Part model, mm, in its own coordinate system. A direction names the side the tool comes from. Round coordinates to 2 decimals unless told otherwise and drop trailing zeros. Write each loop counter-clockwise with the first axis right and the second up, starting at its lowest first coordinate (ties: lowest second). Pieces come first, ordered by that corner, then holes. Notation, with made-up numbers: (-14, -6.5) -> (1, -6.5) arc R21 ccw to (1, 23.5) -> close; hole circle Ø8 at (70, 79). An arc over 180 degrees is marked (long way). Return JSON: item names as keys, results as strings. Group by question number.
```python
from build123d import *

# Parameters (mm, degrees)
SZKIC4_R                    = 75
DODANIE_WYCI_GNI_CIE2_DEPTH = 14
SZKIC5_R                    = 23.5
WYTNIJ_WYCI_GNI_CIE3_DEPTH  = 12
SZKIC6_R                    = 13
WYTNIJ_WYCI_GNI_CIE4_DEPTH  = 12
SZKIC7_R                    = 75
SZKIC7_R_2                  = 72.5
WYTNIJ_WYCI_GNI_CIE5_DEPTH  = 10
SZKIC8_R                    = 1.5
WYTNIJ_WYCI_GNI_CIE6_DEPTH  = 6
SZKIC10_R                   = 1.5
WYTNIJ_WYCI_GNI_CIE7_DEPTH  = 6
SZYK_KO_OWY1_COUNT          = 4


with BuildPart() as part:
    # Szkic4 → Dodanie-wyciągnięcie2 (new body)
    with BuildSketch(Plane(origin=(0, 0, 0), x_dir=(1, 0, 0), z_dir=(0, 1, 0))):
        Circle(SZKIC4_R)
    extrude(amount=DODANIE_WYCI_GNI_CIE2_DEPTH)

    # Szkic5 → Wytnij-wyciągnięcie3 (cut)
    with BuildSketch(Plane(origin=(0, 14, 0), x_dir=(1, 0, 0), z_dir=(0, 1, 0))):
        Circle(SZKIC5_R)
    extrude(amount=-WYTNIJ_WYCI_GNI_CIE3_DEPTH, mode=Mode.SUBTRACT)

    # Szkic6 → Wytnij-wyciągnięcie4 (cut)
    with BuildSketch(Plane(origin=(0, 2, 0), x_dir=(1, 0, 0), z_dir=(0, 1, 0))):
        Circle(SZKIC6_R)
    extrude(amount=-WYTNIJ_WYCI_GNI_CIE4_DEPTH, mode=Mode.SUBTRACT)

    # Szkic7 → Wytnij-wyciągnięcie5 (cut)
    with BuildSketch(Plane.XZ):
        Circle(SZKIC7_R)
        Circle(SZKIC7_R_2, mode=Mode.SUBTRACT)
    extrude(amount=-WYTNIJ_WYCI_GNI_CIE5_DEPTH, mode=Mode.SUBTRACT)

    # Szkic8 → Wytnij-wyciągnięcie6 (cut)
    with BuildSketch(Plane(origin=(0, 0, 0), x_dir=(-1, 0, 0), z_dir=(0, -1, 0))):
        with Locations((23.060270904, -19.500356556)):
            Circle(SZKIC8_R)
        with Locations((-28.863517887, 24.407731054)):
            Circle(SZKIC8_R)
    extrude(amount=-WYTNIJ_WYCI_GNI_CIE6_DEPTH, mode=Mode.SUBTRACT)

    # Szkic10 → Wytnij-wyciągnięcie7 (cut)
    with BuildSketch(Plane(origin=(0, 0, 72.5), x_dir=(0, -1, 0), z_dir=(0, 0, -1))):
        with Locations((-6, 6)):
            Circle(SZKIC10_R)
    wytnij_wyci_gni_cie7 = extrude(amount=WYTNIJ_WYCI_GNI_CIE7_DEPTH, mode=Mode.SUBTRACT)

    # Szyk kołowy1: Wytnij-wyciągnięcie7 ×4 about axis
    szyk_ko_owy1_axis = Axis((0, 0, 0), (0, 1, 0))
    for i in range(1, SZYK_KO_OWY1_COUNT):
        add(wytnij_wyci_gni_cie7.rotate(szyk_ko_owy1_axis, i * 360 / SZYK_KO_OWY1_COUNT), mode=Mode.SUBTRACT)


solid = part.part
```
Item 1: Wall check: L1, parallel to X at y = 5.25, z = -1; L2, parallel to Y at x = 67, z = -31; L3, parallel to Z at x = -1, y = 12.5. Give the ranges that are in metal, low to high.
Item 2: Two-plate mould, pull along X, no slides. Class faces 1 (the face through (-10.316, 1.014, 7.91)), 2 (the face through (69.15, 4.93, 21.78)), 3 (the face through (-39.2, 10, 61.5)): released by +X, released by -X, zero draft, split by the parting line, or undercut.
Item 3: Cut at B-B (z = 0). Write the cut outline in (x, y), then the cut area to 3 significant figures.
Item 4: Flat gauge pins, fed straight in: P1, Ø2.5, axis at y = 6, z = 6, coming from the -X side; P2, Ø5, axis at y = 9, z = 26.5, coming from the +X side; P3, Ø8, axis at x = 13, z = -10.5, coming from the +Y side. Where does each tip first touch, or does it go through?
Item 5: Cut at C-C (z = -28). Write the cut outline in (x, y), then the cut area to 3 significant figures.
Item 6: Which spindle directions (+Z, -Z, +X, -X, +Y, -Y) get a long thin tool onto all of the face, cutting with end or side? Do faces 4 (the face through (22.4, 8.1, -7.1)), 5 (the face through (16, 14, -18)). Say none if no direction does.
Item 7: Cut at D-D (x = 44). Write the cut outline in (y, z), then the cut area to 3 significant figures.
Item 8: Cut at A-A (x = 0). Write the cut outline in (y, z), then the cut area to 3 significant figures.
Checks:
{
 "1": {"L1": "x = -72.49 to -23.48, 23.48 to 72.49", "L2": "y = 10 to 14", "L3": "z = -74.99 to -23.48, 23.48 to 74.99"},
 "2": {"face 1": "undercut", "face 2": "split by the parting line", "face 3": "zero draft"},
 "3": {"outline": "(-75, 10) -> (-72.5, 10) -> (-72.5, 0) -> (-13, 0) -> (-13, 2) -> (-23.5, 2) -> (-23.5, 14) -> (-75, 14) -> close; (13, 0) -> (72.5, 0) -> (72.5, 10) -> (75, 10) -> (75, 14) -> (23.5, 14) -> (23.5, 2) -> (13, 2) -> close", "area": "1,430 mm2"},
 "4": {"P1": "stops at x = -72.34", "P2": "stops at x = 70.99", "P3": "stops at y = 2"},
 "5": {"outline": "(-69.58, 10) -> (-66.87, 10) -> (-66.87, 0) -> (66.87, 0) -> (66.87, 10) -> (69.58, 10) -> (69.58, 14) -> (-69.58, 14) -> close", "area": "1,890 mm2"},
 "6": {"face 4": "+Y", "face 5": "+Z, -Z, +X, -X, +Y"},
 "7": {"outline": "(0, -57.62) -> (10, -57.62) -> (10, -60.74) -> (14, -60.74) -> (14, 60.74) -> (10, 60.74) -> (10, 57.62) -> (0, 57.62) -> close", "area": "1,640 mm2"},
 "8": {"outline": "(0, -72.5) -> (10, -72.5) -> (10, -75) -> (14, -75) -> (14, -23.5) -> (2, -23.5) -> (2, -13) -> (0, -13) -> close; (0, 13) -> (2, 13) -> (2, 23.5) -> (14, 23.5) -> (14, 75) -> (10, 75) -> (10, 72.5) -> (0, 72.5) -> close", "area": "1,430 mm2"}
}
